The model under review builds one solid part; all positions refer to its coordinate system, in mm. A direction names the side the tool comes from. Coordinates: 2 decimals unless noted, no trailing zeros. Write each loop counter-clockwise with the first axis right and the second up, starting at its lowest first coordinate (ties: lowest second). Pieces come first, ordered by that corner, then holes.
```python
from build123d import *

# Parameters (mm, degrees)
BOSS_EXTRUDE4_DEPTH     = 1.5875
M3_CLEARANCE_HOLE3_D    = 3
M3_CLEARANCE_HOLE1_D    = 3.1
M3_CLEARANCE_HOLE4_D    = 2.95
M3_CLEARANCE_HOLE2_D    = 3.1
BOSS_EXTRUDE6_DEPTH     = 3.175
FILLET1_R               = 2
FILLET3_R               = 1
CUT_EXTRUDE4_DEPTH      = 121.250075508
CUT_EXTRUDE4_DEPTH_BACK = 121.250075508
SKETCH27_OUTSIDE_W      = 217.324
SKETCH27_OUTSIDE_H      = 197.151
SKETCH27_OUTSIDE_W_2    = 94
SKETCH27_OUTSIDE_H_2    = 40


with BuildPart() as part:
    # Sketch1 → Boss-Extrude4 (new, symmetric)
    with BuildSketch(Plane(origin=(0, 0, 0), x_dir=(1, 0, 0), z_dir=(0, 1, 0))):
        with BuildLine():
            Line((-62.799553621, 32.496136604), (-73.969425011, 32.691107434))
            Line((-73.969425011, 32.691107434), (-77.053684287, 35.88495141))
            ThreePointArc((-77.053684287, 35.88495141), (-84.36642289, 10.358894189), (-83.446216027, -16.178041625))
            Line((-83.446216027, -16.178041625), (-79.680911643, -13.825218315))
            Line((-79.680911643, -13.825218315), (-69.484649137, -16.179210996))
            Line((-69.484649137, -16.179210996), (-43.894490772, -57.132025032))
            Line((-43.894490772, -57.132025032), (-43.894490772, -64.826600275))
            Line((-43.894490772, -64.826600275), (-43.094490772, -64.826600275))
            Line((-43.094490772, -64.826600275), (-34, -64.826600275))
            Line((-34, -64.826600275), (-34, -55.55))
            Line((-34, -55.55), (-34, -53.55))
            Line((-34, -53.55), (-20, -53.55))
            Line((-20, -53.55), (-19.718918331, -55.55))
            Line((-19.718918331, -55.55), (19.718918331, -55.55))
            Line((19.718918331, -55.55), (20, -53.55))
            Line((20, -53.55), (34, -53.55))
            Line((34, -53.55), (34, -55.55))
            Line((34, -55.55), (34, -64.826600275))
            Line((34, -64.826600275), (43.094490772, -64.826600275))
            Line((43.094490772, -64.826600275), (43.894490772, -64.826600275))
            Line((43.894490772, -64.826600275), (43.894490772, -57.132025032))
            Line((43.894490772, -57.132025032), (69.484649137, -16.179210996))
            Line((69.484649137, -16.179210996), (79.680911643, -13.825218315))
            Line((79.680911643, -13.825218315), (83.446216027, -16.178041625))
            ThreePointArc((83.446216027, -16.178041625), (84.610662337, -8.126242604), (85, 0))
            ThreePointArc((85, 0), (82.98964744, 18.377116688), (77.053684287, 35.88495141))
            Line((77.053684287, 35.88495141), (73.969425011, 32.691107434))
            Line((73.969425011, 32.691107434), (62.799553621, 32.496136604))
            Line((62.799553621, 32.496136604), (30.284668021, 63.895396642))
            Line((30.284668021, 63.895396642), (30.089697191, 75.065268032))
            Line((30.089697191, 75.065268032), (33.173956467, 78.259112008))
            ThreePointArc((33.173956467, 78.259112008), (0, 85), (-33.173956467, 78.259112008))
            Line((-33.173956467, 78.259112008), (-30.089697191, 75.065268032))
            Line((-30.089697191, 75.065268032), (-30.284668021, 63.895396642))
            Line((-30.284668021, 63.895396642), (-62.799553621, 32.496136604))
        make_face()
    extrude(amount=BOSS_EXTRUDE4_DEPTH, both=True)

    # M3 Clearance Hole3 (through all)
    with Locations(Plane(origin=(0, -1.5875, 0), x_dir=(-1, 0, 0), z_dir=(0, -1, 0))):
        with Locations((36.5, -50), (36.5, -38), (-36.5, -50), (-36.5, -38)):
            Hole(M3_CLEARANCE_HOLE3_D / 2)

    # M3 Clearance Hole1 (through all)
    with Locations(Plane(origin=(0, 1.5875, 0), x_dir=(1, 0, 0), z_dir=(0, 1, 0))):
        with Locations((-78.542321426, -8.49139241), (78.542321426, -8.49139241), (74.155025063, 27.240269049), (-74.155025063, 27.240269049)):
            Hole(M3_CLEARANCE_HOLE1_D / 2)

    # M3 Clearance Hole4 (through all)
    with Locations(Plane(origin=(0, -1.5875, 0), x_dir=(-1, 0, 0), z_dir=(0, -1, 0))):
        with Locations((-67.099301622, -15.278865202), (-50.141885166, -42.416404279), (-61.062544382, 30.698137949), (-38.043670771, 52.927205804), (50.141885166, -42.416404279), (67.099301622, -15.278865202), (38.043670771, 52.927205804), (61.062544382, 30.698137949)):
            Hole(M3_CLEARANCE_HOLE4_D / 2)

    # M3 Clearance Hole2 (through all)
    with Locations(Plane(origin=(0, 1.5875, 0), x_dir=(1, 0, 0), z_dir=(0, 1, 0))):
        with Locations((27, 76.497766718), (-27, 76.497766718)):
            Hole(M3_CLEARANCE_HOLE2_D / 2)

    # Sketch22 → Boss-Extrude6 (add)
    with BuildSketch(Plane(origin=(0, 1.5875, 0), x_dir=(1, 0, 0), z_dir=(0, 1, 0))):
        Polygon((65.061950694, 32.535626892), (30.245177733, 66.157793715), (30.284668021, 63.895396642), (62.799553621, 32.496136604), align=None)
        Polygon((-30.284668021, 63.895396642), (-30.245177733, 66.157793715), (-65.061950694, 32.535626892), (-62.799553621, 32.496136604), align=None)
        Polygon((43.894490772, -60.151352895), (71.689396914, -15.670204865), (69.484649137, -16.179210996), (43.894490772, -57.132025032), align=None)
        Polygon((-69.484649137, -16.179210996), (-71.689396914, -15.670204865), (-43.894490772, -60.151352895), (-43.894490772, -57.132025032), align=None)
    extrude(amount=-BOSS_EXTRUDE6_DEPTH)

    # Fillet1
    fillet1_edges = [part.edges().sort_by_distance(p)[0] for p in [
        (-30.245177733, -0.79375, -66.157793715),
        (-65.061950694, -0.79375, -32.535626892),
        (-71.689396914, -0.79375, 15.670204865),
        (-43.894490772, -0.79375, 60.151352895),
        (43.894490772, 0.79375, 60.151352895),
        (71.689396914, 0.79375, 15.670204865),
        (65.061950694, -0.79375, -32.535626892),
        (30.245177733, 0.79375, -66.157793715),
        (30.089697191, -0.79375, -75.065268032),
        (73.969425011, -0.79375, -32.691107434),
        (79.680911643, -0.79375, 13.825218315),
        (-79.680911643, -0.79375, 13.825218315),
        (-73.969425011, -0.79375, -32.691107434),
        (-30.089697191, -0.79375, -75.065268032),
    ]]
    fillet(fillet1_edges, radius=FILLET1_R)

    # Fillet3
    fillet3_edges = [part.edges().sort_by_distance(p)[0] for p in [
        (33.173956467, -0.79375, -78.259112008),
        (77.053684287, 0.79375, -35.88495141),
        (83.446216027, -0.79375, 16.178041625),
        (43.894490772, -0.79375, 64.826600275),
        (34, 0.79375, 64.826600275),
        (34, -0.79375, 53.55),
        (20, -0.79375, 53.55),
        (19.718918331, 0.79375, 55.55),
        (-19.718918331, 0.79375, 55.55),
        (-20, -0.79375, 53.55),
        (-34, -0.79375, 53.55),
        (-34, 0.79375, 64.826600275),
        (-43.894490772, -0.79375, 64.826600275),
        (-83.446216027, -0.79375, 16.178041625),
        (-77.053684287, -0.79375, -35.88495141),
        (-33.173956467, -0.79375, -78.259112008),
    ]]
    fillet(fillet3_edges, radius=FILLET3_R)

    # Sketch27 outside → Cut-Extrude4 (cut, two sides: drawn at the far end of the back side and taken through both)
    with BuildSketch(Plane(origin=(0, 1.5875, 0), x_dir=(1, 0, 0), z_dir=(0, 1, 0)).offset(-CUT_EXTRUDE4_DEPTH_BACK)):
        with Locations((0, 10.0865)):
            Rectangle(SKETCH27_OUTSIDE_W, SKETCH27_OUTSIDE_H)
        with Locations((0, -47.826600275)):
            Rectangle(SKETCH27_OUTSIDE_W_2, SKETCH27_OUTSIDE_H_2, mode=Mode.SUBTRACT)
    extrude(amount=CUT_EXTRUDE4_DEPTH + CUT_EXTRUDE4_DEPTH_BACK, mode=Mode.SUBTRACT)


solid = part.part
```
Item 1: Take a section at A-A, the plane z = 38. Write out the cut boundary in (x, y).
Solved:
outline: (-47, -1.59) - (-38, -1.59) - (-38, 1.59) - (-47, 1.59) - close; (-35, -1.59) - (35, -1.59) - (35, 1.59) - (-35, 1.59) - close; (38, -1.59) - (47, -1.59) - (47, 1.59) - (38, 1.59) - close
Item 2: To check wall thickness, follow line 1 along X through (y, z) = (0.95, 38); line 2 along Z through (x, y) = (-36.5, -0.15); line 3 along X through (y, z) = (0.1, 50.5). State the ranges of each line that lie inside material, in increasing order.
Solved:
line 1: x = -47 to -38, -35 to 35, 38 to 47
line 2: z = 27.83 to 36.5, 39.5 to 48.5, 51.5 to 64.83
line 3: x = -47 to -37.91, -35.09 to 35.09, 37.91 to 47
Item 3: Machinability: for faces 4 (the face through (43.894, 0, 62)), 5 (the face through (-43.894, 0, 62)), 6 (the face through (27, 0, 53.55)), 7 (the face through (-47, 0, 42)), which of the approach directions +Z, -Z, +X, -X, +Y, -Y give a long, thin tool a straight path to every point of the face, cutting with its end or side? Answer none if there is none.
Solved:
face 4: +Z, +X, +Y, -Y
face 5: +Z, -X, +Y, -Y
face 6: +Z, +Y, -Y
face 7: +Z, -Z, -X, +Y, -Y
Item 4: Take a section at C-C, the plane x = 36.5. Write out the cut boundary in (y, z), plus the area to 3 significant figures.
Solved:
outline: (-1.59, 27.83) - (1.59, 27.83) - (1.59, 36.5) - (-1.59, 36.5) - close; (-1.59, 39.5) - (1.59, 39.5) - (1.59, 48.5) - (-1.59, 48.5) - close; (-1.59, 51.5) - (1.59, 51.5) - (1.59, 64.83) - (-1.59, 64.83) - close
area: 98.4 mm2
Item 5: For pin 1 (1.6 mm diameter, centred on y = 0.5, z = 60.5, fed in from +X); pin 2 (1.8 mm diameter, centred on x = 36.5, z = 50, fed in from +Y); pin 3 (1.6 mm diameter, centred on y = 0.5, z = 61.5, fed in from +X); pin 4 (1 mm diameter, centred on x = -5, y = 0.5, fed in from +Z), all flat-tipped, find the tip position at first contact; note any pin that passes through.
Solved:
pin 1: stops at x = 44.18
pin 2: passes through
pin 3: stops at x = 43.89
pin 4: stops at z = 55.55
Item 6: Take a section at B-B, the plane y = 0. Count the separate pieces of the cut face and the enclosed holes in it, plus the area to 3 significant figures.
Solved:
separate pieces: 1
enclosed holes: 4
area: 2,720 mm2
Item 7: Take a section at D-D, the plane z = 58. Write out the cut boundary in (x, y).
Solved:
outline: (-45.24, -1.59) - (-34, -1.59) - (-34, 1.59) - (-45.24, 1.59) - close; (34, -1.59) - (45.24, -1.59) - (45.24, 1.59) - (34, 1.59) - close
Item 8: Mouldability with a two-part tool opening along X and no side actions: class faces 1 (the face through (34, 0, 59)), 2 (the face through (45.58, 0.022, 57.455)), 3 (the face through (-1, -1.588, 42)) as pulls with the +X half, pulls with the -X half, needs draft (parallel to the pull), parting line crosses it, or undercut.
Solved:
face 1: undercut
face 2: pulls with the +X half
face 3: needs draft
